For this review, use the dimensioned drawing (mm, ordinates from the lowest corner) and the shaded views. A direction names the side the tool comes from. Round coordinates to 2 decimals unless told otherwise and drop trailing zeros. Write each loop counter-clockwise with the first axis right and the second up, starting at its lowest first coordinate (ties: lowest second). Pieces come first, ordered by that corner, then holes. Notation, with made-up numbers: (87.25, -9) - (145.25, -9) arc R19 cw to (145.25, 20) - close; hole circle Ø1 at (47.25, 74.5). An arc over 180 degrees is marked (long way). Return JSON: item names as keys, results as strings.
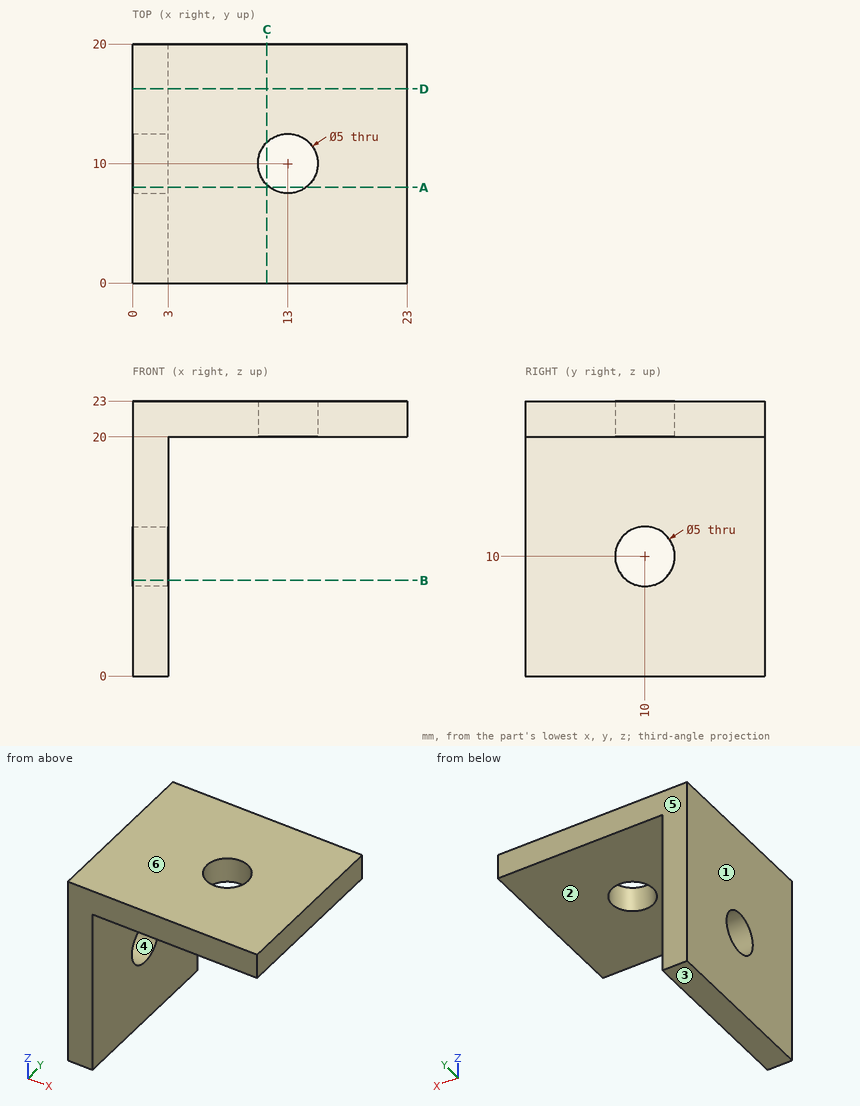
(1) Mouldability with a two-part tool opening along Z and no side actions: class the marked faces 3, 4, 5 and 6 as released by +Z, released by -Z, zero draft, split by the parting line, or undercut.
Filled in:
{"face 3": "released by -Z", "face 4": "undercut", "face 5": "zero draft", "face 6": "released by +Z"}
(2) Add section B-B (z = 8). Write out the cut boundary in (x, y).
Filled in:
{"outline": "(0, 0) - (3, 0) - (3, 8.5) - (0, 8.5) - close; (0, 11.5) - (3, 11.5) - (3, 20) - (0, 20) - close"}
(3) Wall thickness on line 1 (X direction, y = 10, z = 20.7); line 2 (Y direction, x = 0.9, z = 10); line 3 (X direction, y = 7.75, z = 6.75): over which ranges is each line inside the solid? List them lowest first.
Filled in:
{"line 1": "x = 0 to 10.5, 15.5 to 23", "line 2": "y = 0 to 7.5, 12.5 to 20", "line 3": "x = 0 to 3"}
(4) Add section A-A (y = 8). Write out the cut boundary in (x, z).
Filled in:
{"outline": "(0, 0) - (3, 0) - (3, 8.5) - (0, 8.5) - close; (0, 11.5) - (3, 11.5) - (3, 20) - (11.5, 20) - (11.5, 23) - (0, 23) - close; (14.5, 20) - (23, 20) - (23, 23) - (14.5, 23) - close"}
(5) Clearance check with flat-ended pins moving along their axes: pin 1 Ø8 at (y, z) = (6, 15) entering from +X; pin 2 Ø10 at (x, y) = (13, 7) entering from -Z. State where each tip first meets the part, or that it passes through.
Filled in:
{"pin 1": "stops at x = 3", "pin 2": "stops at z = 20"}
(6) Add section D-D (y = 16.25). Write out the cut boundary in (x, z), plus the area to 3 significant figures.
Filled in:
{"outline": "(0, 0) - (3, 0) - (3, 20) - (23, 20) - (23, 23) - (0, 23) - close", "area": "129 mm2"}
(7) Add section C-C (x = 11.25). Write out the cut boundary in (y, z), plus the area to 3 significant figures.
Filled in:
{"outline": "(0, 20) - (8.21, 20) - (8.21, 23) - (0, 23) - close; (11.79, 20) - (20, 20) - (20, 23) - (11.79, 23) - close", "area": "49.3 mm2"}
(8) For the marked faces 1 and 2, list the 3-axis set-ups (+Z, -Z, +X, -X, +Y, -Y) from which the entire face can be reached by the end or side of a thin tool; tool diameter is ignored.
Filled in:
{"face 1": "+Z, -Z, -X, +Y, -Y", "face 2": "-Z, +X, +Y, -Y"}
